from build123d import *

# Parameters (mm, degrees)
SKETCH1_R           = 7.575
BOSS_EXTRUDE1_DEPTH = 5.2
CUT_EXTRUDE1_DEPTH  = 3.6
BOSS_EXTRUDE2_DEPTH = 18.9
FILLET1_R           = 1
BOSS_EXTRUDE3_DEPTH = 4.85
SKETCH6_R           = 1.875
BOSS_EXTRUDE4_DEPTH = 2.55
CUT_EXTRUDE2_DEPTH  = 4
SKETCH7_R           = 7.575
BOSS_EXTRUDE5_DEPTH = 2.8


with BuildPart() as part:
    # Sketch1 → Boss-Extrude1 (new body)
    with BuildSketch(Plane(origin=(0, 0, 0), x_dir=(1, 0, 0), z_dir=(0, 1, 0))):
        Circle(SKETCH1_R)
    extrude(amount=BOSS_EXTRUDE1_DEPTH)

    # Sketch2 → Cut-Extrude1 (cut)
    with BuildSketch(Plane.XZ):
        with BuildLine():
            Line((-4.359330502, -1.388114754), (0, -4.575))
            ThreePointArc((0, -4.575), (2.7, 3.693321676), (-4.359330502, -1.388114754))
        make_face()
    extrude(amount=-CUT_EXTRUDE1_DEPTH, mode=Mode.SUBTRACT)

    # Sketch4 → Boss-Extrude2 (add)
    with BuildSketch(Plane(origin=(0, 5.2, 0), x_dir=(1, 0, 0), z_dir=(0, 1, 0))):
        Polygon((6.611448404, 0), (0, 6.611448404), (-6.611448404, 0), (0, -6.611448404), align=None)
        Polygon((4.242640687, 0), (0, 4.242640687), (-4.242640687, 0), (0, -4.242640687), align=None, mode=Mode.SUBTRACT)
    extrude(amount=BOSS_EXTRUDE2_DEPTH)

    # Fillet1
    fillet1_edges = [part.edges().sort_by_distance(p)[0] for p in [
        (3.305724202, 24.1, 3.305724202),
        (3.305724202, 24.1, -3.305724202),
        (-3.305724202, 24.1, -3.305724202),
        (-3.305724202, 24.1, 3.305724202),
        (0, 14.65, 6.611448404),
        (6.611448404, 14.65, 0),
        (0, 14.65, -6.611448404),
        (-6.611448404, 14.65, 0),
    ]]
    fillet(fillet1_edges, radius=FILLET1_R)

    # Sketch5 → Boss-Extrude3 (add)
    with BuildSketch(Plane(origin=(0, 5.2, 0), x_dir=(1, 0, 0), z_dir=(0, 1, 0))):
        Polygon((0, -4.242640687), (4.242640687, 0), (0, 4.242640687), (-4.242640687, 0), align=None)
    extrude(amount=BOSS_EXTRUDE3_DEPTH)

    # Sketch6 → Boss-Extrude4 (add)
    with BuildSketch(Plane(origin=(0, 10.05, 0), x_dir=(1, 0, 0), z_dir=(0, 1, 0))):
        Circle(SKETCH6_R)
    extrude(amount=BOSS_EXTRUDE4_DEPTH)

    # Sketch3 → Cut-Extrude2 (cut)
    with BuildSketch(Plane.XZ.offset(-3.6)):
        with BuildLine():
            Line((-1.9, 2.157689737), (1.9, 2.157689737))
            ThreePointArc((1.9, 2.157689737), (0, -2.875), (-1.9, 2.157689737))
        make_face()
    extrude(amount=-CUT_EXTRUDE2_DEPTH, mode=Mode.SUBTRACT)

    # Sketch7 → Boss-Extrude5 (add)
    with BuildSketch(Plane(origin=(0, 5.2, 0), x_dir=(1, 0, 0), z_dir=(0, 1, 0))):
        Circle(SKETCH7_R)
        with BuildLine():
            Line((-5.904341623, -0.707106781), (-0.707106781, -5.904341623))
            ThreePointArc((-0.707106781, -5.904341623), (0, -6.197234842), (0.707106781, -5.904341623))
            Line((0.707106781, -5.904341623), (5.904341623, -0.707106781))
            ThreePointArc((5.904341623, -0.707106781), (6.197234842, 0), (5.904341623, 0.707106781))
            Line((5.904341623, 0.707106781), (0.707106781, 5.904341623))
            ThreePointArc((0.707106781, 5.904341623), (0, 6.197234842), (-0.707106781, 5.904341623))
            Line((-0.707106781, 5.904341623), (-5.904341623, 0.707106781))
            ThreePointArc((-5.904341623, 0.707106781), (-6.197234842, 0), (-5.904341623, -0.707106781))
        make_face(mode=Mode.SUBTRACT)
    extrude(amount=BOSS_EXTRUDE5_DEPTH)


solid = part.part
The model under review builds one solid part; all positions refer to its coordinate system, in mm. A direction names the side the tool comes from. Give positions to 0.01 mm unless a question says otherwise; leave off trailing zeros. Order: outer loops, then holes, each group sorted by start corner. A loop starts at its lowest first (then second) coordinate and runs counter-clockwise, first axis right, second up. Notation, with made-up numbers: M 40,25.5 L 44,25.5 A23 cw 44,53.5 Z; hole C -23.75,6 d7. An arc over 180 degrees is marked long. One line per question, with ' | ' between items. Start each with the question number.
1) Mouldability with a two-part tool opening along Z and no side actions: class faces 5 (the face through (-3.07, 23.8, 3.14)), 6 (the face through (0.011, 15.656, -6.197)), 7 (the face through (2.09, 16.98, 2.15)), 8 (the face through (-1.8, 0, -3.5)) as pulls with the +Z half, pulls with the -Z half, needs draft (parallel to the pull), parting line crosses it, or undercut.
2) Consider section A-A, the plane y = 12. Give the boundary of the cut face in (x, z) (3 decimals), then the cut area to 3 significant figures.
3) Consider section C-C, the plane y = 2. Give the boundary of the cut face in (x, z) (3 decimals).
4) Clearance check with flat-ended pins moving along their axes: P1, Ø1.5, axis at x = 0, y = 14, coming from the +Z side; P2, Ø5, axis at x = 4.5, z = 5.5, coming from the -Y side; P3, Ø1.5, axis at x = 3.5, y = 20.5, coming from the +Z side; P4, Ø1.5, axis at x = -1, z = -1.5, coming from the -Y side. State where each tip first meets the part, or that it passes through.
5) Consider section B-B, the plane y = 17. Give the boundary of the cut face in (x, z).
6) Wall thickness on L1, parallel to X at y = 2.65, z = 0 (3 decimals); L2, parallel to Y at x = -5.75, z = 4.5; L3, parallel to Y at x = -3.25, z = 0.75: over which ranges is each line inside the solid? List them lowest first. Write a range as from..to.
7) For faces 1 (the face through (-3.34, 15.44, 3.27)), 2 (the face through (-3.5, 8, -3.5)), 3 (the face through (3.34, 15.44, -3.27)), 4 (the face through (-0.011, 15.656, 6.197)), list the 3-axis set-ups (+Z, -Z, +X, -X, +Y, -Y) from which the entire face can be reached by the end or side of a thin tool; tool diameter is ignored.
Found:
1) face 5: pulls with the +Z half | face 6: pulls with the -Z half | face 7: undercut | face 8: needs draft
2) outline: M -5.904,-0.707 L -0.707,-5.904 A1 ccw 0.707,-5.904 L 5.904,-0.707 A1 ccw 5.904,0.707 L 0.707,5.904 A1 ccw -0.707,5.904 L -5.904,0.707 A1 ccw Z; C 0,0 d3.75; hole M -4.243,0 L 0,-4.243 L 4.243,0 L 0,4.243 Z | area: 61.6 mm²
3) outline: C 0,0 d15.15; hole M -4.359,-1.388 L 0,-4.575 A4.575 ccw long Z
4) P1: stops at z = 6.2 | P2: stops at y = 0 | P3: stops at z = 3.86 | P4: stops at y = 7.6
5) outline: M -5.9,-0.71 L -0.71,-5.9 A1 ccw 0.71,-5.9 L 5.9,-0.71 A1 ccw 5.9,0.71 L 0.71,5.9 A1 ccw -0.71,5.9 L -5.9,0.71 A1 ccw Z; hole M -4.24,0 L 0,-4.24 L 4.24,0 L 0,4.24 Z
6) L1: x = -7.575..-4.575, 4.575..7.575 | L2: y = 0..8 | L3: y = 3.6..10.05
7) face 1: +Z, -X, +Y | face 2: +Y | face 3: -Z, +X, +Y | face 4: +Z, +Y
